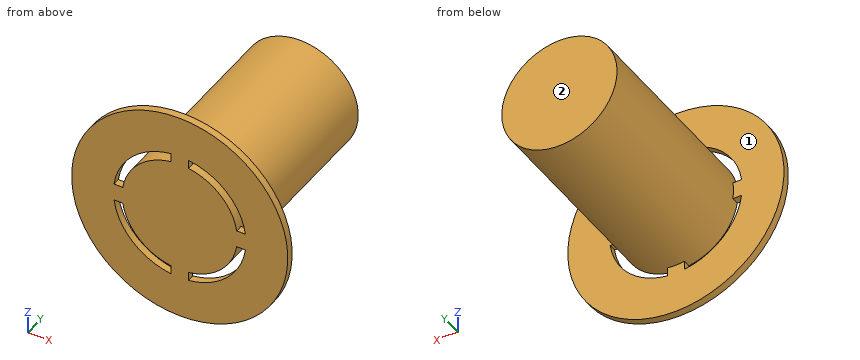
```python
from build123d import *

# Parameters (mm, degrees)
SKETCH1_R           = 4
BOSS_EXTRUDE1_DEPTH = 13.75
SKETCH2_R           = 7.5
SKETCH2_R_2         = 4.6
BOSS_EXTRUDE2_DEPTH = 0.5
BOSS_EXTRUDE3_DEPTH = 0.5


with BuildPart() as part:
    # Sketch1 → Boss-Extrude1 (new body)
    with BuildSketch(Plane(origin=(0, 0, 0), x_dir=(1, 0, 0), z_dir=(0, 1, 0))):
        with Locations(Location((0, 0, 0), (0, 0, 270))):
            Circle(SKETCH1_R)
    extrude(amount=BOSS_EXTRUDE1_DEPTH)



with BuildPart() as body_2:
    # Sketch2 → Boss-Extrude2 (new body)
    with BuildSketch(Plane(origin=(0, 0, 0), x_dir=(-1, 0, 0), z_dir=(0, -1, 0))):
        with Locations(Location((0, 0, 0), (0, 0, 90))):
            Circle(SKETCH2_R)
        with Locations(Location((0, 0, 0), (0, 0, 90))):
            Circle(SKETCH2_R_2, mode=Mode.SUBTRACT)
    extrude(amount=-BOSS_EXTRUDE2_DEPTH)


with BuildPart() as part_1:
    add(part.part)

    add(body_2.part)  # Boss-Extrude3 merges body 2
    # Sketch3 → Boss-Extrude3 (add)
    with BuildSketch(Plane(origin=(0, 0, 0), x_dir=(-1, 0, 0), z_dir=(0, -1, 0))):
        with BuildLine():
            ThreePointArc((4.5607017, -0.6), (4.6, 0), (4.5607017, 0.6))
            Line((4.5607017, 0.6), (3.954743987, 0.6))
            ThreePointArc((3.954743987, 0.6), (4, 0), (3.954743987, -0.6))
            Line((3.954743987, -0.6), (4.5607017, -0.6))
        make_face()
        with BuildLine():
            Line((0.6, 3.954743987), (0.6, 4.5607017))
            ThreePointArc((0.6, 4.5607017), (0, 4.6), (-0.6, 4.5607017))
            Line((-0.6, 4.5607017), (-0.6, 3.954743987))
            ThreePointArc((-0.6, 3.954743987), (0, 4), (0.6, 3.954743987))
        make_face()
        with BuildLine():
            ThreePointArc((-0.6, -4.5607017), (0, -4.6), (0.6, -4.5607017))
            Line((0.6, -4.5607017), (0.6, -3.954743987))
            ThreePointArc((0.6, -3.954743987), (0, -4), (-0.6, -3.954743987))
            Line((-0.6, -3.954743987), (-0.6, -4.5607017))
        make_face()
        with BuildLine():
            Line((-3.954743987, 0.6), (-4.5607017, 0.6))
            ThreePointArc((-4.5607017, 0.6), (-4.6, 0), (-4.5607017, -0.6))
            Line((-4.5607017, -0.6), (-3.954743987, -0.6))
            ThreePointArc((-3.954743987, -0.6), (-4, 0), (-3.954743987, 0.6))
        make_face()
    extrude(amount=-BOSS_EXTRUDE3_DEPTH)


solid = part_1.part
```
The model under review builds one solid part; all positions refer to its coordinate system, in mm. Face numbers are marked on the shaded views. A direction names the side the tool comes from. Round coordinates to 2 decimals unless told otherwise and drop trailing zeros. Write each loop counter-clockwise with the first axis right and the second up, starting at its lowest first coordinate (ties: lowest second). Pieces come first, ordered by that corner, then holes.
(1) Wall thickness on L1, parallel to Y at x = 4.25, z = 2.5; L2, parallel to Z at x = 0, y = 9.25; L3, parallel to X at y = 10, z = -3.5: over which ranges is each line inside the solid? List them lowest first.
(2) We need section A-A on z = 0. Give the boundary of the cut face in (x, y), and give its area (4 significant figures).
(3) We need section B-B on x = 3.5. Give the boundary of the cut face in (y, z), and give its area (3 significant figures).
(4) Insertion check: pin 1 (1 mm diameter, centred on x = -5.5, z = -1.5, fed in from +Y); pin 2 (0.6 mm diameter, centred on x = 4.5, y = 0.5, fed in from +Z); pin 3 (5 mm diameter, centred on y = 7.5, z = 1, fed in from -X). Each pin has a flat end and moves straight along its axis. Give the tip position at first contact, or say it passes through.
(5) We need section D-D on x = 0. Give the boundary of the cut face in (y, z), and give its area (4 significant figures).
(6) We need section C-C on z = 3. Give the boundary of the cut face in (x, y).
(7) Machinability: for the marked faces 1 and 2, which of the approach directions +Z, -Z, +X, -X, +Y, -Y give a long, thin tool a straight path to every point of the face, cutting with its end or side? Answer none if there is none.
Findings below:
1. L1: y = 0 to 0.5
1. L2: z = -4 to 4
1. L3: x = -1.94 to 1.94
2. outline: (-7.5, 0) - (7.5, 0) - (7.5, 0.5) - (4, 0.5) - (4, 13.75) - (-4, 13.75) - (-4, 0.5) - (-7.5, 0.5) - close
2. area: 113.5 mm2
3. outline: (0, -6.63) - (0.5, -6.63) - (0.5, -2.98) - (0, -2.98) - close; (0, -1.94) - (13.75, -1.94) - (13.75, 1.94) - (0, 1.94) - close; (0, 2.98) - (0.5, 2.98) - (0.5, 6.63) - (0, 6.63) - close
3. area: 56.9 mm2
4. pin 1: stops at y = 0.5
4. pin 2: stops at z = 6.21
4. pin 3: stops at x = -4
5. outline: (0, -7.5) - (0.5, -7.5) - (0.5, -4) - (13.75, -4) - (13.75, 4) - (0.5, 4) - (0.5, 7.5) - (0, 7.5) - close
5. area: 113.5 mm2
6. outline: (-6.87, 0) - (-3.49, 0) - (-3.49, 0.5) - (-6.87, 0.5) - close; (-2.65, 0) - (2.65, 0) - (2.65, 13.75) - (-2.65, 13.75) - close; (3.49, 0) - (6.87, 0) - (6.87, 0.5) - (3.49, 0.5) - close
7. face 1: +Y
7. face 2: +Z, -Z, +X, -X, +Y
